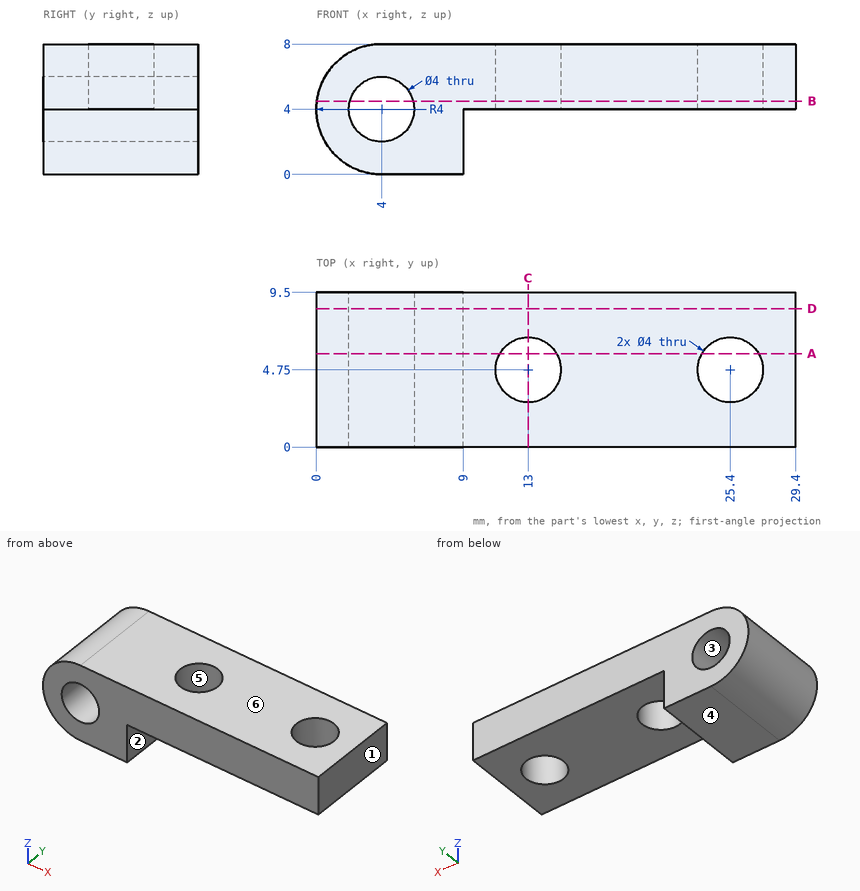
The figure shows three views and two pictorial views of one solid part (mm, origin at its lowest corner). Answer the questions. A direction names the side the tool comes from. Round coordinates to 2 decimals unless told otherwise and drop trailing zeros. Write each loop counter-clockwise with the first axis right and the second up, starting at its lowest first coordinate (ties: lowest second). Pieces come first, ordered by that corner, then holes. Notation, with made-up numbers: M -33,56 L 14,56 A17 cw 14,76 Z; hole C -9,-30.75 d9. An arc over 180 degrees is marked long. Use a Markdown table: item, result.
1) The part is cut by section C-C (x = 13). Write down the section's boundary in (y, z).
Answers follow:
| item | result |
|---|---|
| outline | M 0,4 L 2.75,4 L 2.75,8 L 0,8 Z; M 6.75,4 L 9.5,4 L 9.5,8 L 6.75,8 Z |
2) A tool of negligible diameter and unlimited length cuts with its end or side. For the marked faces 1 and 2, from which of +Z, -Z, +X, -X, +Y, -Y can it reach the whole face along a straight path? Write none if from no direction.
Answers follow:
| item | result |
|---|---|
| face 1 | +Z, -Z, +X, +Y, -Y |
| face 2 | -Z, +X, +Y, -Y |
3) The part is cut by section B-B (z = 4.5). Write down the section's boundary in (x, y).
Answers follow:
| item | result |
|---|---|
| outline | M 0.03,0 L 2.06,0 L 2.06,9.5 L 0.03,9.5 Z; M 5.94,0 L 29.4,0 L 29.4,9.5 L 5.94,9.5 Z; hole C 13,4.75 d4; hole C 25.4,4.75 d4 |
4) The part is cut by section D-D (y = 8.5). Write down the section's boundary in (x, z).
Answers follow:
| item | result |
|---|---|
| outline | M 4,0 L 9,0 L 9,4 L 29.4,4 L 29.4,8 L 4,8 A4 ccw Z; hole C 4,4 d4 |
5) The part is cut by section A-A (y = 5.75). Write down the section's boundary in (x, z), plus the area to 3 significant figures.
Answers follow:
| item | result |
|---|---|
| outline | M 4,0 L 9,0 L 9,4 L 11.27,4 L 11.27,8 L 4,8 A4 ccw Z; M 14.73,4 L 23.67,4 L 23.67,8 L 14.73,8 Z; M 27.13,4 L 29.4,4 L 29.4,8 L 27.13,8 Z; hole C 4,4 d4 |
| area | 106 mm2 |
6) Straight lines are drawn through the part: line 1 along Z through (x, y) = (4, 7.5); line 2 along Z through (x, y) = (23, 7.75); line 3 along Z through (x, y) = (2.25, 8). For each, find the intervals that lie inside material, in ascending order. Write a range as [from, to].
Answers follow:
| item | result |
|---|---|
| line 1 | z = [0, 2], [6, 8] |
| line 2 | z = [4, 8] |
| line 3 | z = [0.4, 3.03], [4.97, 7.6] |
7) Flat-ended cylindrical pins translate along their axes: pin 1 (3 mm diameter, centred on y = 4, z = 7, fed in from -X); pin 2 (4.5 mm diameter, centred on y = 6.5, z = 1, fed in from +X); pin 3 (5 mm diameter, centred on x = 19.5, y = 3, fed in from -Z). Find the tip coordinate at first contact, or state that the pin passes through.
Answers follow:
| item | result |
|---|---|
| pin 1 | stops at x = 0.29 |
| pin 2 | stops at x = 9 |
| pin 3 | stops at z = 4 |
8) For a pull along Z with two mould halves and no side action, classify the marked faces 3, 4, 5 and 6 as pulls with the +Z half, pulls with the -Z half, needs draft (parallel to the pull), parting line crosses it, or undercut.
Answers follow:
| item | result |
|---|---|
| face 3 | undercut |
| face 4 | pulls with the -Z half |
| face 5 | needs draft |
| face 6 | pulls with the +Z half |
